CAD build for the part. Positions are in the model's coordinates, mm. Face numbers are marked on the shaded views. Coordinates: 2 decimals unless noted, no trailing zeros. Write each loop counter-clockwise with the first axis right and the second up, starting at its lowest first coordinate (ties: lowest second). Pieces come first, ordered by that corner, then holes. Notation, with made-up numbers: (-12.5, 31) - (20.5, 31) arc R7 ccw to (20.5, 39) - close; hole circle Ø9 at (20, -11). An arc over 180 degrees is marked (long way). Answer in a Markdown table with one row per item. Add a question column.
Q1. Pin check, flat tips, straight feed: pin 1 (10 mm diameter, centred on x = 13.5, z = -13.5, fed in from +Y); pin 2 (3 mm diameter, centred on x = -10, z = -8, fed in from -Y); pin 3 (1.6 mm diameter, centred on x = -2, y = 12, fed in from -Z). Stop position of each tip, or through.
Q2. Band-saw the part on D-D (z = -11.5). List the corners of the cut face in (x, y).
Q3. Band-saw the part on B-B (y = 0). List the corners of the cut face in (x, z).
Q4. Band-saw the part on C-C (x = -3). List the corners of the cut face in (y, z), and give its area (3 significant figures).
Q5. Two-plate mould, pull along Y, no slides. Class the marked faces 1, 2 and 3: +Y half, -Y half, draft (parallel to the pull), parting line (faces both ways), or undercut.
Q6. Drill centre lines: line 1 along Y through (x, z) = (-33, 0); line 2 along Z through (x, y) = (6.5, -6); line 3 along Y through (x, z) = (-38, 8). Where is each one in solid material? Low to high. Write a range as from..to.
Q7. Band-saw the part on A-A (z = 0). List the corners of the cut face in (x, y), and give its area (3 significant figures).
```python
from build123d import *

# Parameters (mm, degrees)
IZIM1_R                     = 25
IZIM1_R_2                   = 10
Y_KSEKLIK_EKSTR_ZYON1_DEPTH = 80.5
IZIM3_W                     = 6
IZIM3_H                     = 5.6
KES_EKSTR_ZYON1_DEPTH       = 80.5


with BuildPart() as part:
    # Çizim1 → Yükseklik-Ekstrüzyon1 (new, symmetric)
    with BuildSketch(Plane(origin=(0, 0, 0), x_dir=(0, 0, -1), z_dir=(1, 0, 0))):
        Circle(IZIM1_R)
        Circle(IZIM1_R_2, mode=Mode.SUBTRACT)
    extrude(amount=Y_KSEKLIK_EKSTR_ZYON1_DEPTH, both=True)

    # Çizim3 → Kes-Ekstrüzyon1 (cut, symmetric)
    with BuildSketch(Plane(origin=(0, 0, 0), x_dir=(0, 0, -1), z_dir=(1, 0, 0))):
        with Locations((0, 10)):
            Rectangle(IZIM3_W, IZIM3_H)
    extrude(amount=KES_EKSTR_ZYON1_DEPTH, both=True, mode=Mode.SUBTRACT)


solid = part.part
```
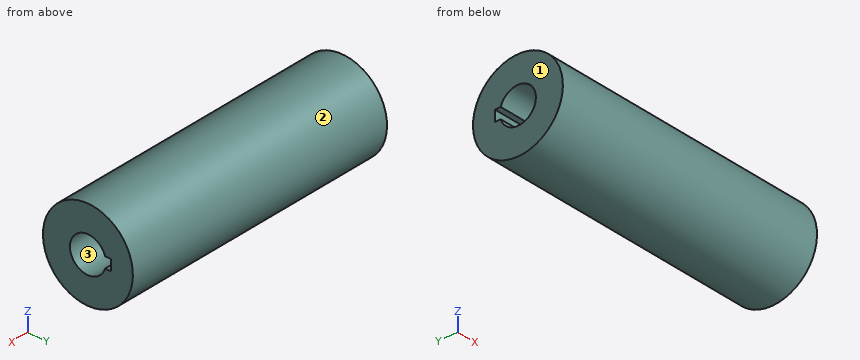
Checked values:
| question | item | result |
|---|---|---|
| 1 | pin 1 | stops at y = 23.51 |
| 1 | pin 2 | stops at y = -24.14 |
| 1 | pin 3 | stops at z = -22.35 |
| 2 | outline | (-80.5, -22.2) - (80.5, -22.2) - (80.5, 22.2) - (-80.5, 22.2) - close |
| 3 | outline | (-80.5, -25) - (80.5, -25) - (80.5, -10) - (-80.5, -10) - close; (-80.5, 10) - (80.5, 10) - (80.5, 25) - (-80.5, 25) - close |
| 4 | outline | circle Ø50 at (0, 0); hole (9.54, -3) - (12.8, -3) - (12.8, 3) - (9.54, 3) arc R10 ccw (long way) to start |
| 4 | area | 1,630 mm² |
| 5 | face 1 | draft |
| 5 | face 2 | parting line |
| 5 | face 3 | undercut |
| 6 | line 1 | y = -25..-10, 12.8..25 |
| 6 | line 2 | z = -24.27..-8, 8..24.27 |
| 6 | line 3 | y = -23.69..-6, 6..23.69 |
| 7 | outline | (-80.5, -25) - (80.5, -25) - (80.5, -10) - (-80.5, -10) - close; (-80.5, 12.8) - (80.5, 12.8) - (80.5, 25) - (-80.5, 25) - close |
| 7 | area | 4,380 mm² |
